Work out the finished part from the listing and answer in its coordinate system (mm). Give positions to 0.01 mm unless a question says otherwise; leave off trailing zeros. Put each result on its own line as item: value.
```python
from build123d import *

# Parameters (mm, degrees)
SKETCH1_W        = 406.4
SKETCH1_H        = 304.8
EXTRUSION1_DEPTH = 9.525
FILLET1_R        = 19.05
FILLET2_R        = 19.05
FILLET3_R        = 19.05
FILLET4_R        = 19.05
HOLE1_D          = 5.842
HOLE1_DEPTH      = 25.4
HOLE1_TIP        = 1.755113868
HOLE4_D          = 5
HOLE4_DEPTH      = 25.4
HOLE4_TIP        = 1.502151548
HOLE5_D          = 4
HOLE5_DEPTH      = 25.4
HOLE5_TIP        = 1.201721238
HOLE6_D          = 11.2
HOLE6_DEPTH      = 6
HOLE7_D          = 9.75
HOLE7_DEPTH      = 5


with BuildPart() as part:
    # Sketch1 → Extrusion1 (new body)
    with BuildSketch(Plane(origin=(0, 0, 0), x_dir=(-1, 0, 0), z_dir=(0, 1, 0))):
        Rectangle(SKETCH1_W, SKETCH1_H)
    extrude(amount=EXTRUSION1_DEPTH)

    # Fillet1
    fillet1_edges = [part.edges().sort_by_distance(p)[0] for p in [
        (203.2, 4.7625, 152.4),
    ]]
    fillet(fillet1_edges, radius=FILLET1_R)

    # Fillet2
    fillet2_edges = [part.edges().sort_by_distance(p)[0] for p in [
        (203.2, 4.7625, -152.4),
    ]]
    fillet(fillet2_edges, radius=FILLET2_R)

    # Fillet3
    fillet3_edges = [part.edges().sort_by_distance(p)[0] for p in [
        (-203.2, 4.7625, 152.4),
    ]]
    fillet(fillet3_edges, radius=FILLET3_R)

    # Fillet4
    fillet4_edges = [part.edges().sort_by_distance(p)[0] for p in [
        (-203.2, 4.7625, -152.4),
    ]]
    fillet(fillet4_edges, radius=FILLET4_R)

    # Hole1
    with Locations(Plane(origin=(0, 9.525, 0), x_dir=(1, 0, 0), z_dir=(0, 1, 0))):
        with Locations((-177.8, -127), (-177.8, -76.2), (-177.8, -25.4), (-177.8, 25.4), (-177.8, 76.2), (-177.8, 127), (-152.4, -127), (-152.4, -76.2), (-152.4, -25.4), (-152.4, 25.4), (-152.4, 76.2), (-152.4, 127), (-127, -127), (-127, -76.2), (-127, -25.4), (-127, 25.4), (-127, 76.2), (-127, 127), (-101.6, -127), (-101.6, -76.2), (-101.6, -25.4), (-101.6, 25.4), (-101.6, 76.2), (-101.6, 127), (-76.2, -127), (-76.2, -76.2), (-76.2, -25.4), (-76.2, 25.4), (-76.2, 76.2), (-76.2, 127), (-50.8, -127), (-50.8, -76.2), (-50.8, -25.4), (-50.8, 25.4), (-50.8, 76.2), (-50.8, 127), (-25.4, -127), (-25.4, -76.2), (-25.4, -25.4), (-25.4, 25.4), (-25.4, 76.2), (-25.4, 127), (0, -127), (0, -76.2), (0, -25.4), (0, 25.4), (0, 76.2), (0, 127), (25.4, -127), (25.4, -76.2), (25.4, -25.4), (25.4, 25.4), (25.4, 76.2), (25.4, 127), (50.8, -127), (50.8, -76.2), (50.8, -25.4), (50.8, 25.4), (50.8, 76.2), (50.8, 127), (76.2, -127), (76.2, -76.2), (76.2, -25.4), (76.2, 25.4), (76.2, 76.2), (76.2, 127)):
            Hole(HOLE1_D / 2, depth=HOLE1_DEPTH)
            with Locations((0, 0, -(HOLE1_DEPTH + HOLE1_TIP / 2))):  # 118° drill point
                Cone(0, HOLE1_D / 2, HOLE1_TIP, mode=Mode.SUBTRACT)

    # Hole4
    with Locations(Plane(origin=(0, 9.525, 0), x_dir=(1, 0, 0), z_dir=(0, 1, 0))):
        with Locations((-147.400000005, 17.5), (-147.400000005, 52.5), (-112.400000005, 52.5), (-112.400000005, -17.5), (-112.400000005, 17.5), (-147.400000005, -17.5), (-147.400000005, -52.5), (-112.400000005, -52.5), (112.400000005, -17.5), (147.400000005, -17.5), (147.400000005, -52.5), (112.400000005, -52.5), (112.400000005, 52.5), (147.400000005, 17.5), (112.400000005, 17.5), (147.400000005, 52.5)):
            Hole(HOLE4_D / 2, depth=HOLE4_DEPTH)
            with Locations((0, 0, -(HOLE4_DEPTH + HOLE4_TIP / 2))):  # 118° drill point
                Cone(0, HOLE4_D / 2, HOLE4_TIP, mode=Mode.SUBTRACT)

    # Hole5
    with Locations(Plane(origin=(0, 9.525, 0), x_dir=(1, 0, 0), z_dir=(0, 1, 0))):
        with Locations((-19, 11), (19, 11), (-19, -11), (19, -11)):
            Hole(HOLE5_D / 2, depth=HOLE5_DEPTH)
            with Locations((0, 0, -(HOLE5_DEPTH + HOLE5_TIP / 2))):  # 118° drill point
                Cone(0, HOLE5_D / 2, HOLE5_TIP, mode=Mode.SUBTRACT)

    # Hole6
    with Locations(Plane(origin=(-147.400000005, 9.525, -52.5), x_dir=(0, 0, -1), z_dir=(0, 1, 0))):
        with Locations((0, 0), (0, -35), (-35, -35), (-35, 0), (-70, 0), (-70, -35), (-105, -35), (-105, 0), (0, -259.800000009), (0, -294.800000009), (-35, -294.800000009), (-35, -259.800000009), (-70, -259.800000009), (-70, -294.800000009), (-105, -294.800000009), (-105, -259.800000009)):
            Hole(HOLE6_D / 2, depth=HOLE6_DEPTH)

    # Hole7
    with Locations(Plane(origin=(-19, 9.525, -11), x_dir=(0, 0, -1), z_dir=(0, 1, 0))):
        with Locations((0, 0), (0, -38), (-22, -38), (-22, 0)):
            Hole(HOLE7_D / 2, depth=HOLE7_DEPTH)


solid = part.part
```
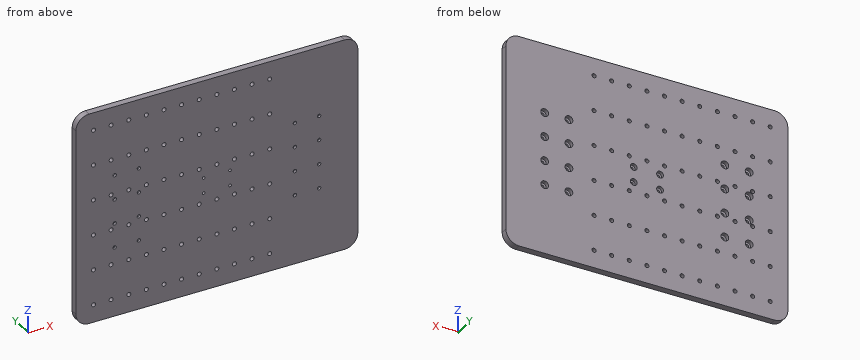
(1) Straight lines are drawn through the part: line 1 (Z direction, x = -147.4, y = 8.2); line 2 (X direction, y = 7.15, z = 17.5); line 3 (X direction, y = 2.7, z = -52.5). For each, find the intervals that lie inside material, in ascending order.
Geometry check:
line 1: z = -152.4 to -58.1, -46.9 to -23.1, -11.9 to 11.9, 23.1 to 46.9, 58.1 to 152.4
line 2: x = -203.2 to -153, -141.8 to -118, -106.8 to 106.8, 118 to 141.8, 153 to 203.2
line 3: x = -203.2 to -149.9, -144.9 to -114.9, -109.9 to 109.9, 114.9 to 144.9, 149.9 to 203.2
(2) Given pin 1 (5.5 mm diameter, centred on x = 147, z = -54.5, fed in from +Y) (3 decimals), flat-ended and moving along its own axis, determine where the tip first touches the part or whether it passes through.
Geometry check:
pin 1: stops at y = 3.525
(3) Section A-A, the plane y = 1.75 is taken. Count the separate pieces of the cut face and the enclosed holes in it, then the cut area to 3 significant figures.
Geometry check:
separate pieces: 1
enclosed holes: 86
area: 121,000 mm²
